Could you check a few things on this model? Use its own coordinates, in mm. Face numbers are marked on the shaded views. A direction names the side the tool comes from. Coordinates: 2 decimals unless noted, no trailing zeros. Loops run counter-clockwise (first coordinate to the right, second up) from the corner with the lowest first, then second, coordinate; pieces in that order, holes last. Notation, with made-up numbers: M 28,68 L 58,68 A27 ccw 58,103 Z; hole C -21,37 d9. An arc over 180 degrees is marked long. Use one line per item in the form item = value. Start each with the question number.
```python
from build123d import *
from OCP.BRepFilletAPI import BRepFilletAPI_MakeChamfer

# Parameters (mm, degrees)
SKETCH1_W                 = 101.6
SKETCH1_H                 = 152.4
BOSS_EXTRUDE1_DEPTH       = 6.35
SKETCH2_W                 = 38.1
SKETCH2_H                 = 63.5
CUT_EXTRUDE1_DEPTH        = 92.800885072
BOSS_EXTRUDE3_DEPTH       = 10.0965
BOSS_EXTRUDE3_DEPTH_BACK  = 6.35
CUT_EXTRUDE2_REACH        = 105.862
SKETCH6_R                 = 3
SKETCH7_W                 = 24.005
SKETCH7_H                 = 2.009
BOSS_EXTRUDE4_DEPTH       = 16.4465
BOSS_EXTRUDE5_REACH       = 129.401
SKETCH10_W                = 13
SKETCH10_H                = 6.35
CUT_EXTRUDE3_REACH        = 138.165
SKETCH11_W                = 13
SKETCH11_H                = 10.0965
BOSS_EXTRUDE6_DEPTH       = 10
CUT_EXTRUDE4_DEPTH        = 2.54
SKETCH14_W                = 101.6
SKETCH14_H                = 6.35
BOSS_EXTRUDE7_DEPTH       = 50.8
SKETCH15_W                = 19.05
SKETCH15_H                = 19.05
BOSS_EXTRUDE8_DEPTH       = 77.47
SKETCH16_W                = 19.05
SKETCH16_H                = 19.05
BOSS_EXTRUDE9_DEPTH       = 6.35
SKETCH17_W                = 184.15
SKETCH17_H                = 83.82
BOSS_EXTRUDE10_DEPTH      = 6.35
BOSS_EXTRUDE11_DEPTH      = 6.35
BOSS_EXTRUDE11_DEPTH_BACK = 6.35
SKETCH18_R                = 19.812
SKETCH18_R_2              = 13.462
SKETCH21_W                = 7.62
SKETCH21_H                = 39.624
BOSS_EXTRUDE13_DEPTH      = 12.7
CHAMFER1_SIZE             = 6.35
CHAMFER1_SIZE_2           = 9.068739843


with BuildPart() as part:
    # Sketch1 → Boss-Extrude1 (new body)
    with BuildSketch(Plane(origin=(0, 0, 0), x_dir=(1, 0, 0), z_dir=(0, 1, 0))):
        Rectangle(SKETCH1_W, SKETCH1_H)
    extrude(amount=-BOSS_EXTRUDE1_DEPTH)

    # Sketch2 → Cut-Extrude1 (cut, through all)
    with BuildSketch(Plane(origin=(0, 0, 0), x_dir=(1, 0, 0), z_dir=(0, 1, 0))):
        Rectangle(SKETCH2_W, SKETCH2_H)
    extrude(amount=-CUT_EXTRUDE1_DEPTH, mode=Mode.SUBTRACT)

    # Sketch4 → Boss-Extrude3 (add, two sides: drawn at the far end of the back side and taken through both)
    with BuildSketch(Plane(origin=(0, 0, 0), x_dir=(1, 0, 0), z_dir=(0, 1, 0)).offset(-BOSS_EXTRUDE3_DEPTH_BACK)):
        Polygon((61.595, -8.509), (50.8, -8.509), (50.8, -14.859), (67.945, -14.859), (67.945, 14.859), (50.8, 14.859), (50.8, 8.509), (61.595, 8.509), align=None)
        Polygon((50.8, -8.509), (21.59, -8.509), (21.59, 8.509), (50.8, 8.509), (50.8, 14.859), (19.05, 14.859), (19.05, -14.859), (50.8, -14.859), align=None)
    extrude(amount=BOSS_EXTRUDE3_DEPTH + BOSS_EXTRUDE3_DEPTH_BACK)

    # Sketch6 → Cut-Extrude2 (cut, up to next)
    with BuildSketch(Plane.ZY.offset(-19.05), mode=Mode.PRIVATE) as cut_extrude2_sk1:
        with Locations((0, 10.0965)):
            Circle(SKETCH6_R)
    cut_extrude2_tool1 = extrude(cut_extrude2_sk1.sketch, amount=-CUT_EXTRUDE2_REACH, mode=Mode.PRIVATE) & part.part
    add(cut_extrude2_tool1.solids().sort_by_distance((19.05, 10.0965, 0))[0], mode=Mode.SUBTRACT)

    # Sketch7 → Boss-Extrude4 (add, through all)
    with BuildSketch(Plane(origin=(0, 10.0965, 0), x_dir=(1, 0, 0), z_dir=(0, 1, 0))):
        with Locations((49.5925, 7.5045)):
            Rectangle(SKETCH7_W, SKETCH7_H)
        with Locations((49.5925, -7.5045)):
            Rectangle(SKETCH7_W, SKETCH7_H)
    extrude(amount=-BOSS_EXTRUDE4_DEPTH)

    # Sketch10 → Boss-Extrude5 (add, up to next)
    with BuildSketch(Plane(origin=(50.8, 0, 0), x_dir=(0, 0, -1), z_dir=(1, 0, 0)), mode=Mode.PRIVATE) as boss_extrude5_sk1:
        with Locations((0, -3.175)):
            Rectangle(SKETCH10_W, SKETCH10_H)
    boss_extrude5_tool1 = extrude(boss_extrude5_sk1.sketch, amount=BOSS_EXTRUDE5_REACH, mode=Mode.PRIVATE) - part.part
    add(boss_extrude5_tool1.solids().sort_by_distance((50.8, -3.175, 0))[0])

    # Sketch11 → Cut-Extrude3 (cut, up to next)
    with BuildSketch(Plane.ZY.offset(-61.595), mode=Mode.PRIVATE) as cut_extrude3_sk1:
        with Locations((0, 5.04825)):
            Rectangle(SKETCH11_W, SKETCH11_H)
    cut_extrude3_tool1 = extrude(cut_extrude3_sk1.sketch, amount=-CUT_EXTRUDE3_REACH, mode=Mode.PRIVATE) & part.part
    add(cut_extrude3_tool1.solids().sort_by_distance((61.595, 5.04825, 0))[0], mode=Mode.SUBTRACT)

    # Sketch12 → Boss-Extrude6 (add)
    with BuildSketch(Plane(origin=(0, 10.0965, 0), x_dir=(1, 0, 0), z_dir=(0, 1, 0))):
        Polygon((67.945, -14.859), (67.945, -6.5), (37.59, -6.5), (37.59, -8.509), (21.59, -8.509), (21.59, -3), (19.05, -3), (19.05, -14.859), align=None)
        Polygon((37.59, 6.5), (67.945, 6.5), (67.945, 14.859), (19.05, 14.859), (19.05, 3), (21.59, 3), (21.59, 8.509), (37.59, 8.509), align=None)
    extrude(amount=BOSS_EXTRUDE6_DEPTH)

    # Sketch13 → Cut-Extrude4 (cut)
    with BuildSketch(Plane.ZY.offset(-19.05)):
        Polygon((3, 10.0965), (7, 10.0965), (7, 14.0965), (11, 14.0965), (11, 17.0965), (7, 17.0965), (7, 20.0965), (3, 20.0965), align=None)
    cut_extrude4 = extrude(amount=-CUT_EXTRUDE4_DEPTH, mode=Mode.SUBTRACT)

    # Mirror1: Cut-Extrude4 across plane
    add(cut_extrude4.mirror(Plane.XY), mode=Mode.SUBTRACT)

    # Sketch14 → Boss-Extrude7 (add)
    with BuildSketch(Plane(origin=(0, 0, -76.2), x_dir=(-1, 0, 0), z_dir=(0, 0, -1))):
        with Locations((0, -3.175)):
            Rectangle(SKETCH14_W, SKETCH14_H)
    extrude(amount=BOSS_EXTRUDE7_DEPTH)

    # Sketch15 → Boss-Extrude8 (add)
    with BuildSketch(Plane.XZ.offset(6.35)):
        with Locations((-60.325, 66.675)):
            Rectangle(SKETCH15_W, SKETCH15_H)
        with Locations((-41.275, -117.475)):
            Rectangle(SKETCH15_W, SKETCH15_H)
    extrude(amount=BOSS_EXTRUDE8_DEPTH)


with BuildPart() as boss_extrude8_piece_1:
    # of the separate pieces the step leaves, piece 1, a body of its own (boss_extrude8_pieces)
    add(part.part.solids().sort_by_distance((-50.8, 0, 76.2))[0])



with BuildPart() as boss_extrude8_piece_2:
    # of the separate pieces the step leaves, piece 2, a body of its own (boss_extrude8_pieces)
    add(part.part.solids().sort_by_distance((-50.8, -83.82, 76.2))[0])


with BuildPart() as boss_extrude8_piece_1_1:
    add(boss_extrude8_piece_1.part)

    add(boss_extrude8_piece_2.part)  # Boss-Extrude9 merges Boss-Extrude8 piece 2
    # Sketch16 → Boss-Extrude9 (add)
    with BuildSketch(Plane(origin=(0, -6.35, 0), x_dir=(1, 0, 0), z_dir=(0, 1, 0))):
        with Locations((-60.325, -66.675)):
            Rectangle(SKETCH16_W, SKETCH16_H)
    extrude(amount=BOSS_EXTRUDE9_DEPTH)

    # Sketch17 → Boss-Extrude10 (add)
    with BuildSketch(Plane.ZY.offset(50.8)):
        with Locations((-34.925, -41.91)):
            Rectangle(SKETCH17_W, SKETCH17_H)
    extrude(amount=BOSS_EXTRUDE10_DEPTH)

    # Sketch18 → Boss-Extrude11 (add, two sides: drawn at the far end of the back side and taken through both)
    # profile 1 of 2: a face of its own
    with BuildSketch(Plane(origin=(0, 0, 0), x_dir=(1, 0, 0), z_dir=(0, 1, 0)).offset(-BOSS_EXTRUDE11_DEPTH_BACK)):
        with Locations(Location((76.2, -76.2, 0), (0, 0, 270))):
            Circle(SKETCH18_R)
        with Locations(Location((76.2, -76.2, 0), (0, 0, 270))):
            Circle(SKETCH18_R_2, mode=Mode.SUBTRACT)
    # profile 2 of 2: a face of its own
    with BuildSketch(Plane(origin=(0, 0, 0), x_dir=(1, 0, 0), z_dir=(0, 1, 0)).offset(-BOSS_EXTRUDE11_DEPTH_BACK)):
        with BuildLine():
            Line((76.2, 96.012), (50.8, 96.012))
            Line((50.8, 96.012), (50.8, 56.388))
            Line((50.8, 56.388), (76.2, 56.388))
            ThreePointArc((76.2, 56.388), (96.012, 76.2), (76.2, 96.012))
        make_face()
        with Locations(Location((76.2, 76.2, 0), (0, 0, 270))):
            Circle(SKETCH18_R_2, mode=Mode.SUBTRACT)
    extrude(amount=BOSS_EXTRUDE11_DEPTH + BOSS_EXTRUDE11_DEPTH_BACK)


with BuildPart() as boss_extrude11_piece_1:
    # of the separate pieces the step leaves, piece 1, a body of its own (boss_extrude11_pieces)
    add(boss_extrude8_piece_1_1.part.solids().sort_by_distance((-50.8, -6.35, 76.2))[0])



with BuildPart() as boss_extrude11_piece_2:
    # of the separate pieces the step leaves, piece 2, a body of its own (boss_extrude11_pieces)
    add(boss_extrude8_piece_1_1.part.solids().sort_by_distance((76.2, 0, 96.012))[0])


with BuildPart() as boss_extrude11_piece_1_1:
    add(boss_extrude11_piece_1.part)

    add(boss_extrude11_piece_2.part)  # Boss-Extrude13 merges Boss-Extrude11 piece 2
    # Sketch21 → Boss-Extrude13 (add)
    with BuildSketch(Plane(origin=(0, 6.35, 0), x_dir=(1, 0, 0), z_dir=(0, 1, 0))):
        with BuildLine():
            Line((56.388, -76.2), (50.8, -76.2))
            Line((50.8, -76.2), (50.8, -57.15))
            Line((50.8, -57.15), (70.758231537, -57.15))
            ThreePointArc((70.758231537, -57.15), (60.383431776, -64.268884645), (56.388, -76.2))
        make_face()
        with Locations((54.61, 76.2)):
            Rectangle(SKETCH21_W, SKETCH21_H)
    extrude(amount=-BOSS_EXTRUDE13_DEPTH)

    # Chamfer1
    chamfer1_edges_1 = [boss_extrude11_piece_1_1.edges().sort_by_distance(p)[0] for p in [
        (50.8, 0, 66.675),
    ]]
    chamfer1_side_1 = [boss_extrude11_piece_1_1.faces().sort_by_distance(p)[0] for p in [
        (50.8, 0.127, 66.675),
    ]]
    chamfer1_edges_2 = [boss_extrude11_piece_1_1.edges().sort_by_distance(p)[0] for p in [
        (50.8, 0, -76.2),
    ]]
    chamfer1_side_2 = [boss_extrude11_piece_1_1.faces().sort_by_distance(p)[0] for p in [
        (50.673, 0, -76.2),
    ]]
    chamfer1 = BRepFilletAPI_MakeChamfer(boss_extrude11_piece_1_1.part.solid().wrapped)
    for e in chamfer1_edges_1:
        chamfer1.Add(CHAMFER1_SIZE - 0.0001, CHAMFER1_SIZE_2 - 0.0001, e.wrapped, chamfer1_side_1[0].wrapped)
    for e in chamfer1_edges_2:
        chamfer1.Add(CHAMFER1_SIZE_2 - 0.0001, CHAMFER1_SIZE - 0.0001, e.wrapped, chamfer1_side_2[0].wrapped)
    add(Compound.cast(chamfer1.Shape()), mode=Mode.REPLACE)  # a hair under: the kernel refuses the full size


solid = boss_extrude11_piece_1_1.part
```
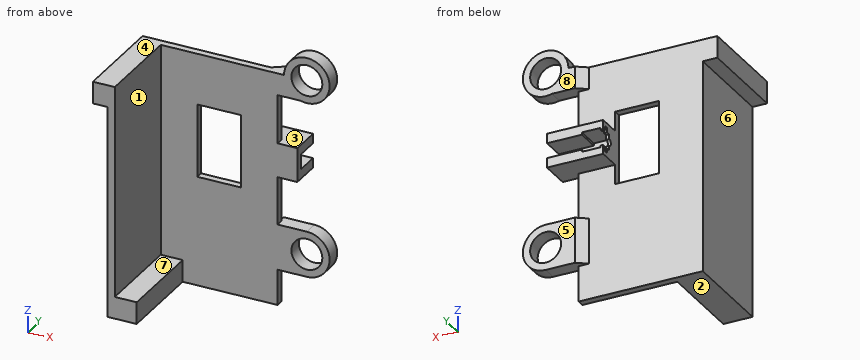
Item 1: I'm going to push flat-ended pins straight in: P1, Ø13, axis at x = 25.5, y = 8, coming from the -Z side; P2, Ø1.5, axis at y = -34, z = 37.5, coming from the +X side; P3, Ø2, axis at y = 9, z = -8, coming from the -X side. Where does each tip first touch, or does it pass through?
Item 2: I want a section at D-D (z = -101.5). Write out the boundary of the cut face in (x, y), plus the area to 3 significant figures.
Item 3: Please list where these lines run through material, in increasing order: line 1 along Z through (x, y) = (71.5, -5); line 2 along Z through (x, y) = (55, 11); line 3 along Y through (x, z) = (35, -106).
Item 4: I want a section at C-C (x = 10.5). Write out the boundary of the cut face in (y, z), plus the area to 3 significant figures.
Item 5: Thinking about a two-plate mould opening in Z: for the marked faces 1, 2 and 3, which applies, pulls with the +Z half, pulls with the -Z half, needs draft (parallel to the pull), parting line crosses it, or undercut?
Item 6: I want a section at B-B (x = 53.5). Write out the boundary of the cut face in (y, z), plus the area to 3 significant figures.
Item 7: For the marked faces 4, 5, 6, 7 and 8, which set-ups out of +Z, -Z, +X, -X, +Y, -Y let a thin tool reach every point of the face, with its end or its side?
Worked answers:
q1.P1 = -14.86
q1.P2 = -50.8
q1.P3 = 19.05
q2.outline = M -57.15,-83.82 L -50.8,-83.82 L -50.8,-6.35 L 50.8,-6.35 L 50.8,0 L -57.15,0 Z
q2.area = 1,180 mm²
q3.line_1 = -96.01 to -88.81, -63.59 to -56.39, 56.95 to 63.59, 88.81 to 95.45
q3.line_2 = -14.86 to -6.5, 6.5 to 14.86
q3.line_3 = -6.35 to 0
q4.outline = M -6.35,-127 L 0,-127 L 0,-31.75 L -6.35,-31.75 Z; M -6.35,31.75 L 0,31.75 L 0,76.2 L -6.35,76.2 Z
q4.area = 887 mm²
q5.face_1 = needs draft
q5.face_2 = pulls with the -Z half
q5.face_3 = undercut
q6.outline = M -6.35,-96.01 L 6.35,-96.01 L 6.35,-56.39 L -6.35,-56.39 Z; M -6.35,-14.86 L 20.1,-14.86 L 20.1,-6.5 L 0,-6.5 L 0,6.5 L 20.1,6.5 L 20.1,14.86 L -6.35,14.86 Z; M -6.35,57.15 L 6.35,57.15 L 6.35,76.2 L -6.35,76.2 Z
q6.area = 1,270 mm²
q7.face_4 = +Z, -X, +Y, -Y
q7.face_5 = -Z, +X, -X, +Y
q7.face_6 = -Z, -X, +Y, -Y
q7.face_7 = +Z, +X, -Y
q7.face_8 = +Z, +X, -X, +Y
